Part model, mm, in its own coordinate system. A direction names the side the tool comes from. Give positions to 0.01 mm unless a question says otherwise; leave off trailing zeros. Write each loop counter-clockwise with the first axis right and the second up, starting at its lowest first coordinate (ties: lowest second). Pieces come first, ordered by that corner, then holes.
```python
from build123d import *

# Parameters (mm, degrees)
CYLINDER001_R     = 9.3
CYLINDER001_DEPTH = 49.5
CYLINDER_R        = 10
CYLINDER_DEPTH    = 50


with BuildPart() as cylinder001:
    # Cylinder001 → Cylinder001 (new body)
    with BuildSketch(Plane.XY.offset(0.5)):
        Circle(CYLINDER001_R)
    extrude(amount=CYLINDER001_DEPTH)


with BuildPart() as cut:
    # Cylinder → Cylinder (new body)
    with BuildSketch(Plane.XY):
        Circle(CYLINDER_R)
    extrude(amount=CYLINDER_DEPTH)

    # Cut: cut Cylinder001
    add(cylinder001.part, mode=Mode.SUBTRACT)


solid = cut.part
```
1) Two-plate mould, pull along X, no slides. Class faces 1 (the face through (-2.17, -9.76, 24.65)), 2 (the face through (0, 0, 0)), 3 (the face through (5, 7.84, 24.9)): +X half, -X half, draft (parallel to the pull), parting line (faces both ways), or undercut.
Answers follow:
face 1: parting line
face 2: draft
face 3: undercut
2) Wall check: L1, parallel to Y at x = 0, z = 46; L2, parallel to Z at x = 5.5, y = -0.5. Give the ranges that are in metal, low to high.
Answers follow:
L1: y = -10 to -9.3, 9.3 to 10
L2: z = 0 to 0.5
3) 3-axis set-ups, long thin cutter, end or side, ignore diameter. For faces 4 (the face through (3, -9, 50)), 5 (the face through (0, 0, 0.5)): which of +Z, -Z, +X, -X, +Y, -Y reach the whole face in a straight line?
Answers follow:
face 4: +Z, +X, -X, +Y, -Y
face 5: +Z
4) Pin check, flat tips, straight feed: pin 1 Ø3 at (x, y) = (-0.5, 1.5) entering from +Z; pin 2 Ø12 at (x, y) = (-3.5, -6.5) entering from +Z; pin 3 Ø3 at (x, z) = (3, 39) entering from -Y; pin 4 Ø1 at (x, z) = (1, 31) entering from -Y. Stop position of each tip, or through.
Answers follow:
pin 1: stops at z = 0.5
pin 2: stops at z = 50
pin 3: stops at y = -9.89
pin 4: stops at y = -9.99
5) Saw through at C-C, the plane z = 46.5. Write the cut outline in (x, y).
Answers follow:
outline: circle Ø20 at (0, 0); hole circle Ø18.6 at (0, 0)
6) Saw through at A-A, the plane x = 0. Write the cut outline in (y, z), then the cut area to 3 significant figures.
Answers follow:
outline: (-10, 0) - (10, 0) - (10, 50) - (9.3, 50) - (9.3, 0.5) - (-9.3, 0.5) - (-9.3, 50) - (-10, 50) - close
area: 79.3 mm2
